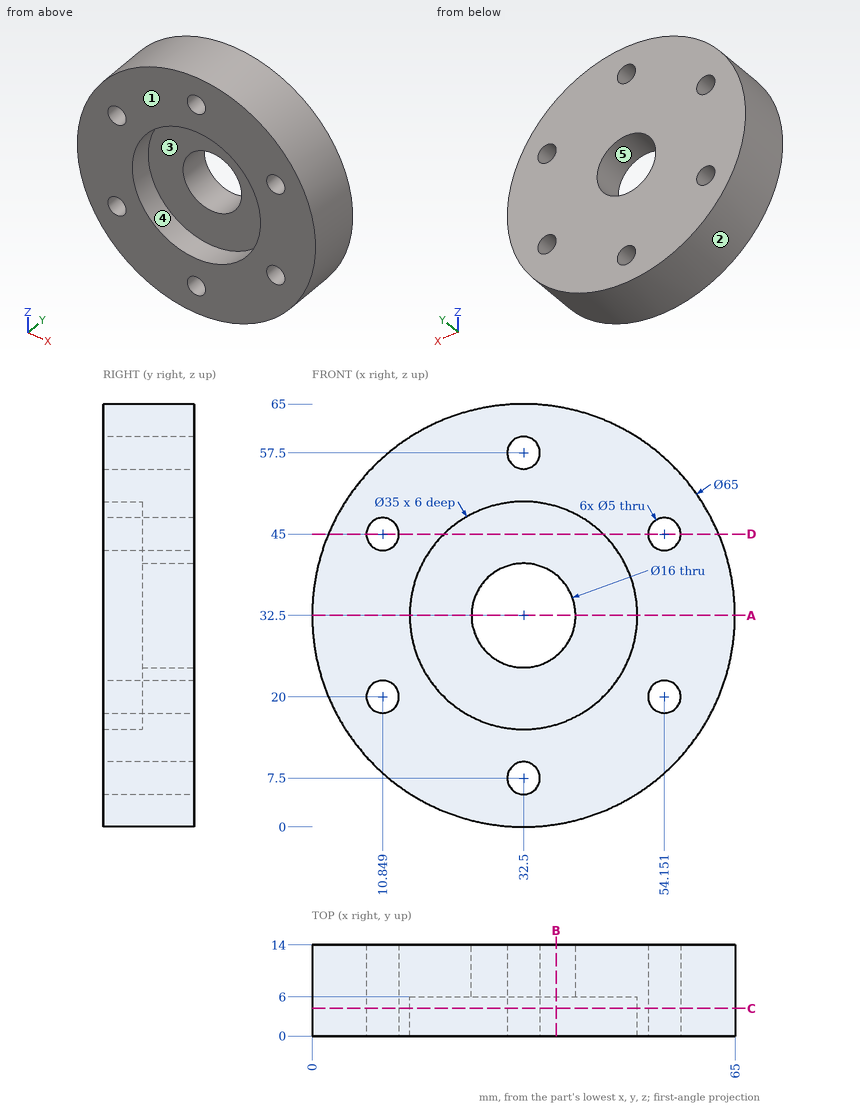
Source: three-view drawing plus pictorial views. Frame: mm from the lowest corner of the part. A direction names the side the tool comes from. Coordinates: 2 decimals unless noted, no trailing zeros. Write each loop counter-clockwise with the first axis right and the second up, starting at its lowest first coordinate (ties: lowest second). Pieces come first, ordered by that corner, then holes. Notation, with made-up numbers: (48, 83) - (54, 83) arc R18 ccw to (54, 115) - close; hole circle Ø5 at (12, -18.5). An arc over 180 degrees is marked (long way). Answer as a JSON object with one key per item and string values.
Q1. Section query A-A, the plane z = 32.5. Output: boundary loops of the cut face in (x, y).
Ans:
{"outline": "(0, 0) - (15, 0) - (15, 6) - (24.5, 6) - (24.5, 14) - (0, 14) - close; (40.5, 6) - (50, 6) - (50, 0) - (65, 0) - (65, 14) - (40.5, 14) - close"}
Q2. Set-up query: the marked faces 4 and 5. Return all of +Z, -Z, +X, -X, +Y, -Y with unobstructed straight access to the full face (end or side cutting, diameter ignored); none if empty.
Ans:
{"face 4": "-Y", "face 5": "+Y, -Y"}
Q3. Material intervals for line 1 (X direction, y = 12, z = 19.5); line 2 (X direction, y = 2.5, z = 21.5); line 3 (Z direction, x = 11.5, y = 12.25) (1 decimal), sorted ascending. Write a range as [from, to].
Ans:
{"line 1": "x = [2.71, 8.4], [13.3, 51.7], [56.6, 62.29]", "line 2": "x = [1.92, 8.85], [12.85, 18.89], [46.11, 52.15], [56.15, 63.08]", "line 3": "z = [7.7, 17.6], [22.4, 42.6], [47.4, 57.3]"}
Q4. First-contact query: pin 1 Ø4 at (x, y) = (7.5, 9.5) entering from +Z; pin 2 Ø6 at (x, z) = (10.85, 45) entering from -Y; pin 3 Ø4 at (x, y) = (13, 3) entering from -Z; pin 4 Ø6 at (y, z) = (5.5, 32.5) entering from +X. Flat tips, straight axial feed; report the tip coordinate or a pass-through.
Ans:
{"pin 1": "stops at z = 55.46", "pin 2": "stops at y = 0", "pin 3": "stops at z = 5.11", "pin 4": "stops at x = 65"}
Q5. Draft query along Z for the marked faces 1, 2 and 3. Return one class per face: released by +Z, released by -Z, zero draft, split by the parting line, or undercut.
Ans:
{"face 1": "zero draft", "face 2": "split by the parting line", "face 3": "undercut"}
Q6. Section query B-B, the plane x = 37.5. Output: boundary loops of the cut face in (y, z) (1 decimal).
Ans:
{"outline": "(0, 0.4) - (14, 0.4) - (14, 26.3) - (6, 26.3) - (6, 15.7) - (0, 15.7) - close; (0, 49.3) - (6, 49.3) - (6, 38.7) - (14, 38.7) - (14, 64.6) - (0, 64.6) - close"}
Q7. Section query C-C, the plane y = 4.25. Output: boundary loops of the cut face in (x, z).
Ans:
{"outline": "circle Ø65 at (32.5, 32.5); hole circle Ø5 at (10.85, 20); hole circle Ø5 at (10.85, 45); hole circle Ø35 at (32.5, 32.5); hole circle Ø5 at (32.5, 7.5); hole circle Ø5 at (32.5, 57.5); hole circle Ø5 at (54.15, 20); hole circle Ø5 at (54.15, 45)"}
Q8. Section query D-D, the plane z = 45. Output: boundary loops of the cut face in (x, y).
Ans:
{"outline": "(2.5, 0) - (8.35, 0) - (8.35, 14) - (2.5, 14) - close; (13.35, 0) - (20.25, 0) - (20.25, 6) - (44.75, 6) - (44.75, 0) - (51.65, 0) - (51.65, 14) - (13.35, 14) - close; (56.65, 0) - (62.5, 0) - (62.5, 14) - (56.65, 14) - close"}
